Geometry: see drawing. Coordinates: mm, zero at the bounding-box minimum. Coordinates: 2 decimals unless noted, no trailing zeros. Loops run counter-clockwise (first coordinate to the right, second up) from the corner with the lowest first, then second, coordinate; pieces in that order, holes last. Notation, with made-up numbers: (65.25, 83.25) - (121.25, 83.25) arc R23 ccw to (121.25, 101.25) - close; hole circle Ø9 at (-34.75, -33). An arc over 180 degrees is marked (long way). Use a Markdown table: item, result. Add a question column.
1. Contact query for flat-ended pins moving along their axis: P1, Ø12, axis at x = 18, y = 32, coming from the -Z side; P2, Ø3, axis at x = 30.5, y = 17, coming from the +Z side; P3, Ø5, axis at x = 13.5, y = 27, coming from the -Z side. Output: stop coordinate, or through.
2. Draft query along X for the marked faces 1, 2 and 3. Return one class per face: released by +X, released by -X, zero draft, split by the parting line, or undercut.
3. Section query A-A on y = 33.5. Return the cut outline in (x, z) (1 decimal).
4. Ray query, L1, parallel to Y at x = 29, z = 17; L2, parallel to X at y = 10, z = 8.5; L3, parallel to X at y = 41, z = 19.5. Return the intervals inside material, ascending. Write a range as [from, to].
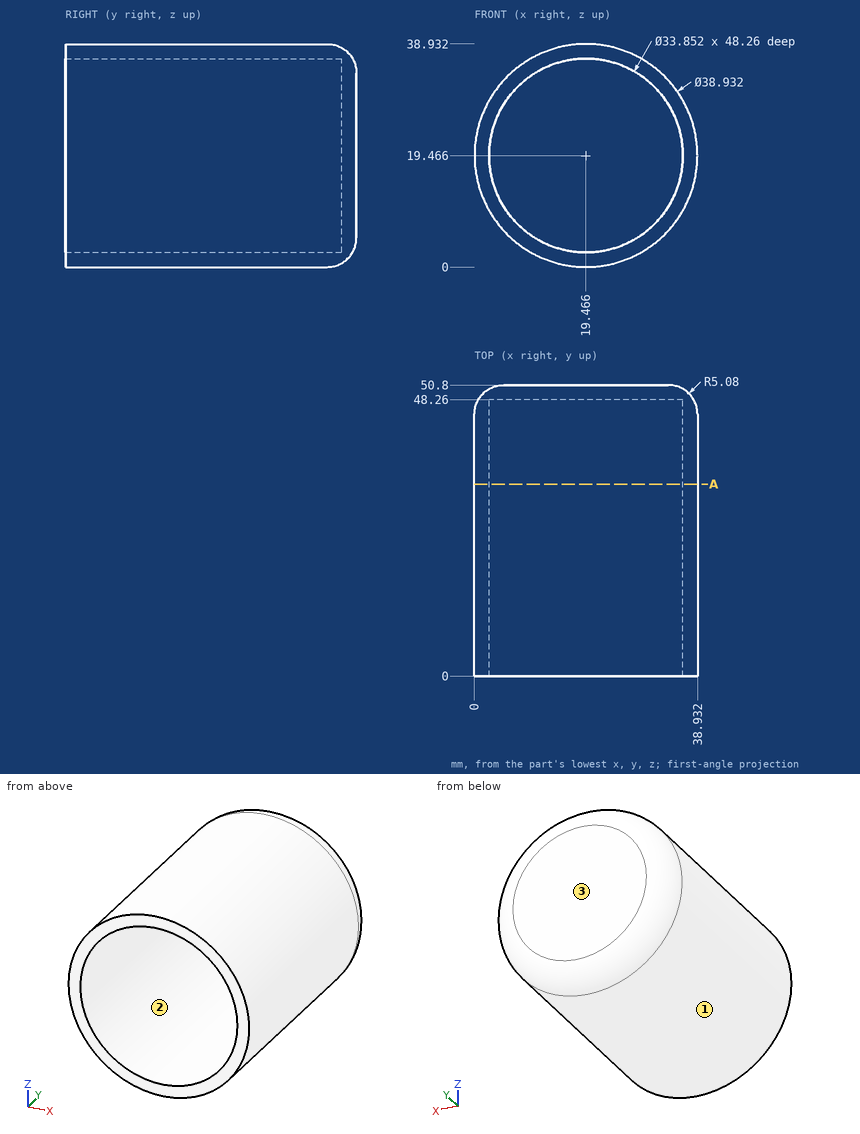
Resolved:
| question | item | result |
|---|---|---|
| 1 | P1 | z = 0 |
| 1 | P2 | z = 36.44 |
| 1 | P3 | z = 0.31 |
| 2 | face 1 | split by the parting line |
| 2 | face 2 | undercut |
| 2 | face 3 | zero draft |
| 3 | outline | circle Ø38.9 at (19.5, 19.5); hole circle Ø33.9 at (19.5, 19.5) |
| 4 | L1 | [48.26, 50.8] |
| 4 | L2 | [3.38, 6.57], [32.36, 35.55] |
| 4 | L3 | [0, 2.54], [36.39, 38.93] |
